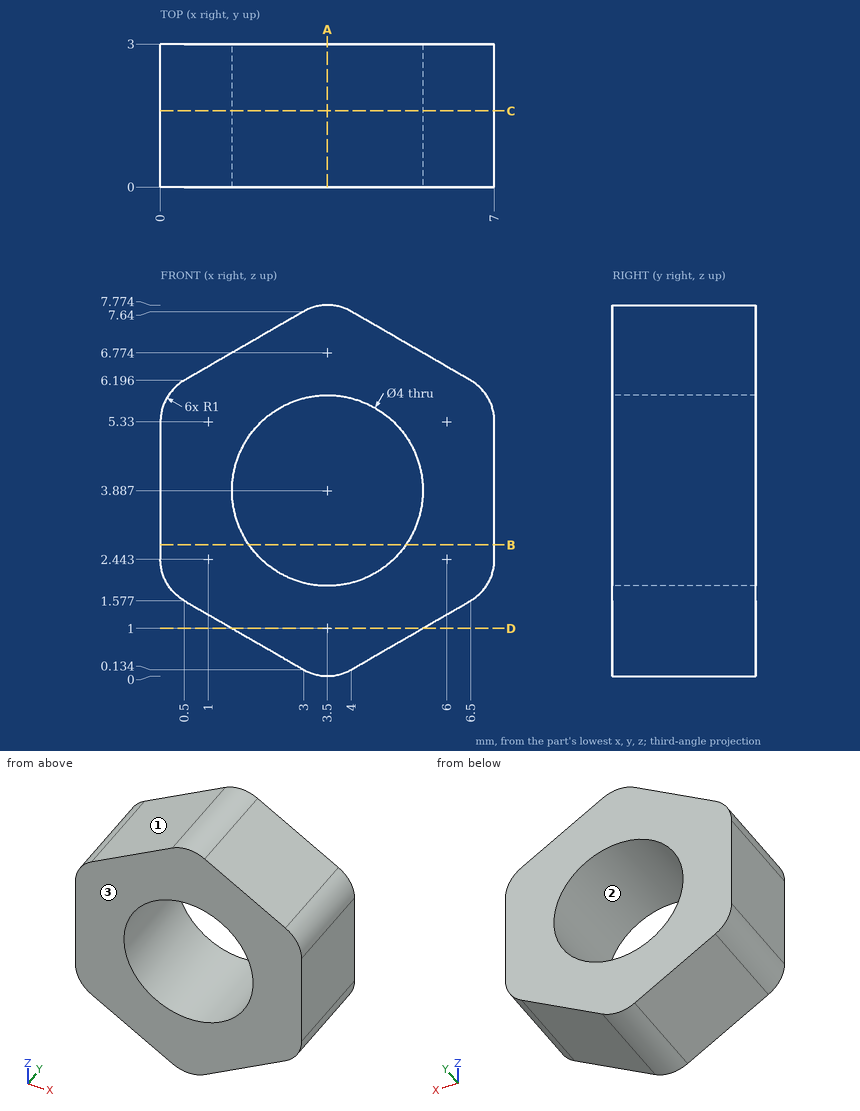
Part print with two shaded views. Sizes in mm from the minimum x, y, z corner. Coordinates: 2 decimals unless noted, no trailing zeros. Write each loop counter-clockwise with the first axis right and the second up, starting at its lowest first coordinate (ties: lowest second). Pieces come first, ordered by that corner, then holes.
(1) Drill centre lines: line 1 (Z direction, x = 3.5, y = 0.9); line 2 (Z direction, x = 0.5, y = 2) (1 decimal); line 3 (X direction, y = 2.25, z = 2.25). Where is each one in solid material? Low to high.
(2) Cut at B-B on z = 2.75. List the corners of the cut face in (x, y) (1 decimal), and give its area (3 significant figures).
(3) Cut at D-D on z = 1. List the corners of the cut face in (x, y), and give its area (3 significant figures).
(4) Cut at C-C on y = 1.6. List the corners of the cut face in (x, z).
(5) Mould opens along Z. For the marked faces 1, 2 and 3 say: pulls with the +Z half, pulls with the -Z half, needs draft (parallel to the pull), parting line crosses it, or undercut.
(6) Cut at A-A on x = 3.5. List the corners of the cut face in (y, z), and give its area (3 significant figures).
Working result:
1. line 1: z = 0 to 1.89, 5.89 to 7.77
1. line 2: z = 1.6 to 6.2
1. line 3: x = 0.02 to 2.35, 4.65 to 6.98
2. outline: (0, 0) - (1.9, 0) - (1.9, 3) - (0, 3) - close; (5.1, 0) - (7, 0) - (7, 3) - (5.1, 3) - close
2. area: 11.1 mm2
3. outline: (1.5, 0) - (5.5, 0) - (5.5, 3) - (1.5, 3) - close
3. area: 12.0 mm2
4. outline: (0, 2.44) arc R1 ccw to (0.5, 1.58) - (3, 0.13) arc R1 ccw to (4, 0.13) - (6.5, 1.58) arc R1 ccw to (7, 2.44) - (7, 5.33) arc R1 ccw to (6.5, 6.2) - (4, 7.64) arc R1 ccw to (3, 7.64) - (0.5, 6.2) arc R1 ccw to (0, 5.33) - close; hole circle Ø4 at (3.5, 3.89)
5. face 1: pulls with the +Z half
5. face 2: undercut
5. face 3: needs draft
6. outline: (0, 0) - (3, 0) - (3, 1.89) - (0, 1.89) - close; (0, 5.89) - (3, 5.89) - (3, 7.77) - (0, 7.77) - close
6. area: 11.3 mm2
